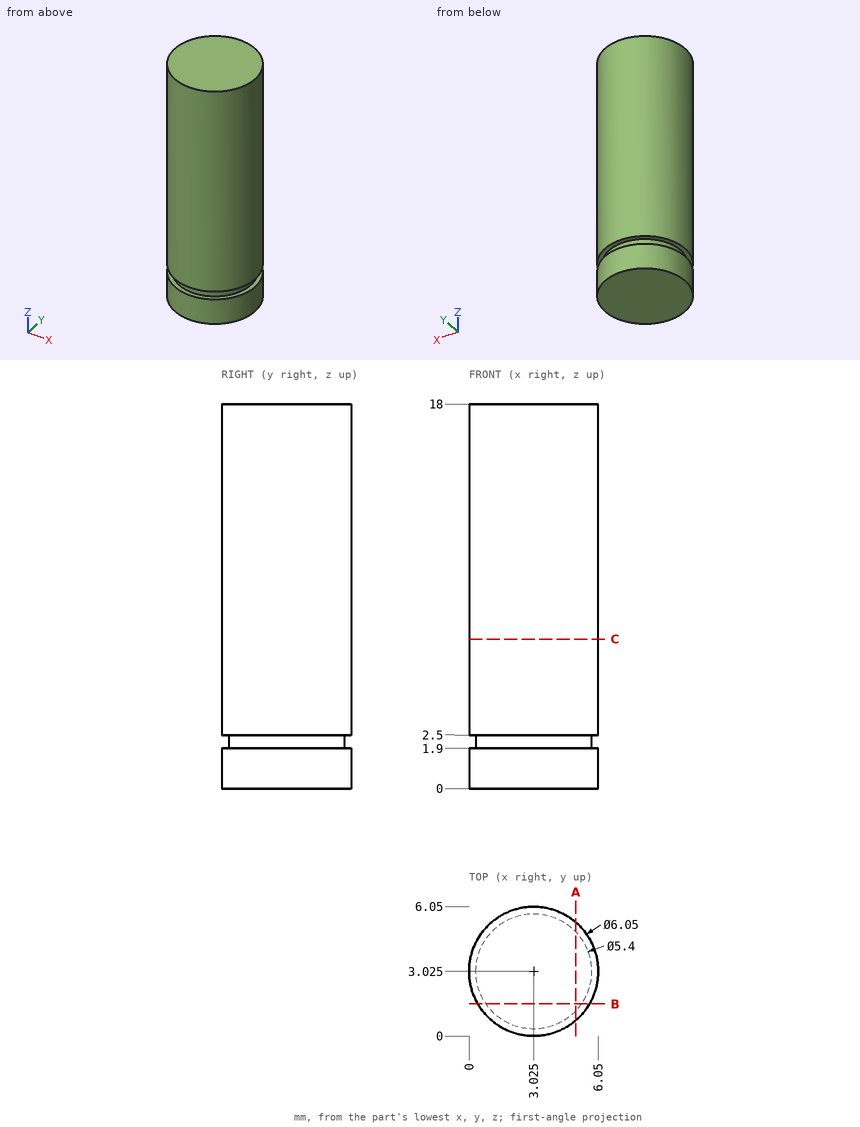
The drawing under review shows one solid part. Ordinate dimensions are in mm from its lowest x, y, z. Coordinates: 2 decimals unless noted, no trailing zeros. Loops run counter-clockwise (first coordinate to the right, second up) from the corner with the lowest first, then second, coordinate; pieces in that order, holes last.
Item 1: Add section A-A (x = 5). Write out the cut boundary in (y, z), and give its area (3 significant figures).
Completed:
outline: (0.73, 0) - (5.32, 0) - (5.32, 1.9) - (4.87, 1.9) - (4.87, 2.5) - (5.32, 2.5) - (5.32, 18) - (0.73, 18) - (0.73, 2.5) - (1.18, 2.5) - (1.18, 1.9) - (0.73, 1.9) - close
area: 81.9 mm2
Item 2: Add section C-C (z = 7). Write out the cut boundary in (x, y) (3 decimals), and give its area (3 significant figures).
Completed:
outline: circle Ø6.05 at (3.025, 3.025)
area: 28.7 mm2
Item 3: Wall thickness on L1, parallel to Z at x = 5.5, y = 4.5; L2, parallel to Y at x = 3.25, z = 6.75; L3, parallel to Y at x = 5.75, z = 9.75: over which ranges is each line inside the solid? List them lowest first.
Completed:
L1: z = 0 to 1.9, 2.5 to 18
L2: y = 0.01 to 6.04
L3: y = 1.71 to 4.34
Item 4: Clearance check with a flat-ended pin moving along its axis: pin 1 (1.5 mm diameter, centred on y = 1.5, z = 13, fed in from -X). State where the tip first meets the part, or that it passes through.
Completed:
pin 1: stops at x = 0.1
Item 5: Add section B-B (y = 1.5). Write out the cut boundary in (x, z), and give its area (3 significant figures).
Completed:
outline: (0.41, 0) - (5.64, 0) - (5.64, 1.9) - (5.25, 1.9) - (5.25, 2.5) - (5.64, 2.5) - (5.64, 18) - (0.41, 18) - (0.41, 2.5) - (0.8, 2.5) - (0.8, 1.9) - (0.41, 1.9) - close
area: 93.6 mm2
